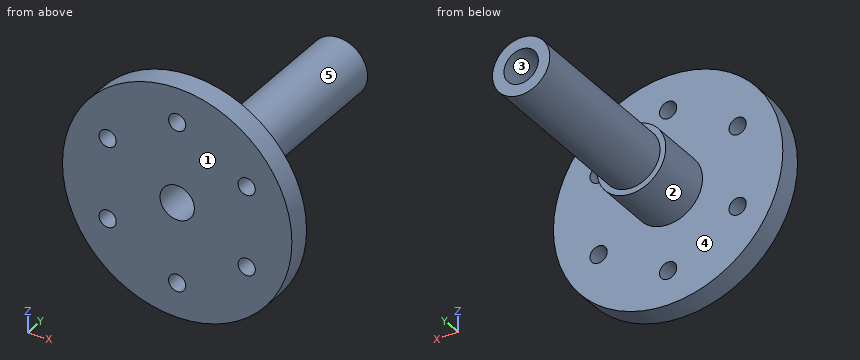
```python
from build123d import *

# Parameters (mm, degrees)
SKETCH_1_R      = 20
SKETCH_1_R_2    = 1.5
SKETCH_1_R_3    = 3
EXTRUDE_1_DEPTH = 4
SKETCH_2_R      = 6
SKETCH_2_R_2    = 3
EXTRUDE_2_DEPTH = 10
SKETCH_3_R      = 5
SKETCH_3_R_2    = 3
EXTRUDE_3_DEPTH = 30


with BuildPart() as part:
    # Sketch 1 → Extrude 1 (new body)
    with BuildSketch(Plane(origin=(0, 0, 0), x_dir=(1, 0, 0), z_dir=(0, 1, 0))):
        with Locations(Location((0, 0, 0), (0, 0, 270))):
            Circle(SKETCH_1_R)
        with Locations(Location((0, 14, 0), (0, 0, 270))):
            Circle(SKETCH_1_R_2, mode=Mode.SUBTRACT)
        with Locations(Location((12.124355653, 7, 0), (0, 0, 270))):
            Circle(SKETCH_1_R_2, mode=Mode.SUBTRACT)
        with Locations(Location((12.124355653, -7, 0), (0, 0, 270))):
            Circle(SKETCH_1_R_2, mode=Mode.SUBTRACT)
        with Locations(Location((0, -14, 0), (0, 0, 270))):
            Circle(SKETCH_1_R_2, mode=Mode.SUBTRACT)
        with Locations(Location((-12.124355653, -7, 0), (0, 0, 270))):
            Circle(SKETCH_1_R_2, mode=Mode.SUBTRACT)
        with Locations(Location((-12.124355653, 7, 0), (0, 0, 270))):
            Circle(SKETCH_1_R_2, mode=Mode.SUBTRACT)
        with Locations(Location((0, 0, 0), (0, 0, 270))):
            Circle(SKETCH_1_R_3, mode=Mode.SUBTRACT)
    extrude(amount=EXTRUDE_1_DEPTH)

    # Sketch 2 → Extrude 2 (add)
    with BuildSketch(Plane(origin=(0, 4, 0), x_dir=(1, 0, 0), z_dir=(0, 1, 0))):
        with Locations(Location((0, 0, 0), (0, 0, 270))):
            Circle(SKETCH_2_R)
        with Locations(Location((0, 0, 0), (0, 0, 270))):
            Circle(SKETCH_2_R_2, mode=Mode.SUBTRACT)
    extrude(amount=EXTRUDE_2_DEPTH)

    # Sketch 3 → Extrude 3 (add)
    with BuildSketch(Plane(origin=(0, 14, 0), x_dir=(1, 0, 0), z_dir=(0, 1, 0))):
        with Locations(Location((0, 0, 0), (0, 0, 270))):
            Circle(SKETCH_3_R)
        with Locations(Location((0, 0, 0), (0, 0, 270))):
            Circle(SKETCH_3_R_2, mode=Mode.SUBTRACT)
    extrude(amount=EXTRUDE_3_DEPTH)


solid = part.part
```
Read the model definition and answer for the solid it produces. Units are mm, in the model's axes. Face numbers are marked on the shaded views. A direction names the side the tool comes from. Coordinates: 2 decimals unless noted, no trailing zeros. Write each loop counter-clockwise with the first axis right and the second up, starting at its lowest first coordinate (ties: lowest second). Pieces come first, ordered by that corner, then holes. Notation, with made-up numbers: (-25.5, 5) - (1.5, 5) arc R35 ccw to (1.5, 44) - close; hole circle Ø1 at (10.25, 16). An arc over 180 degrees is marked (long way). Answer as a JSON object with one key per item and string values. Group by question number.
1. A cutting plane is placed at D-D (y = 7). Determine the outline of the cut face in (x, z), plus the area to 3 significant figures.
2. A cutting plane is placed at C-C (z = -7). Determine the outline of the cut face in (x, y) (3 decimals).
3. Which of the six approach directions +Z, -Z, +X, -X, +Y, -Y give full straight-line access (tool end or side, diameter ignored) to the marked faces 1 and 2?
4. Each of these flat-tipped pins is pushed along its axis until it touches: P1, Ø4, axis at x = -12.12, z = -7, coming from the +Y side; P2, Ø10, axis at y = 6, z = 2, coming from the +X side; P3, Ø2.5, axis at x = 12.12, z = 7, coming from the -Y side (3 decimals); P4, Ø1, axis at x = -4, y = 28, coming from the +Z side. Where does it stop, or does it pass through?
5. A cutting plane is placed at A-A (z = 0). Determine the outline of the cut face in (x, y), plus the area to 3 significant figures.
6. A cutting plane is placed at B-B (x = 0). Determine the outline of the cut face in (y, z), plus the area to 3 significant figures.
7. Consider L1, parallel to X at y = 2.75, z = 7 (3 decimals); L2, parallel to Y at x = -4, z = -9; L3, parallel to Y at x = 5, z = -1. Determine where each line is inside the solid, lowest interval first. Write a range as [from, to].
8. The mould has two halves that part along X. Classify the marked faces 3, 4 and 5: +X half, -X half, draft (parallel to the pull), parting line (faces both ways), or undercut.
Worked out:
{
 "1": {"outline": "circle Ø12 at (0, 0); hole circle Ø6 at (0, 0)", "area": "84.8 mm²"},
 "2": {"outline": "(-18.735, 0) - (-13.624, 0) - (-13.624, 4) - (-18.735, 4) - close; (-10.624, 0) - (10.624, 0) - (10.624, 4) - (-10.624, 4) - close; (13.624, 0) - (18.735, 0) - (18.735, 4) - (13.624, 4) - close"},
 "3": {"face 1": "+Z, -Z, +X, -X, -Y", "face 2": "+Y"},
 "4": {"P1": "stops at y = 4", "P2": "stops at x = 20", "P3": "passes through", "P4": "stops at z = 3.57"},
 "5": {"outline": "(-20, 0) - (-3, 0) - (-3, 44) - (-5, 44) - (-5, 14) - (-6, 14) - (-6, 4) - (-20, 4) - close; (3, 0) - (20, 0) - (20, 4) - (6, 4) - (6, 14) - (5, 14) - (5, 44) - (3, 44) - close", "area": "316 mm²"},
 "6": {"outline": "(0, -20) - (4, -20) - (4, -15.5) - (0, -15.5) - close; (0, -12.5) - (4, -12.5) - (4, -6) - (14, -6) - (14, -5) - (44, -5) - (44, -3) - (0, -3) - close; (0, 3) - (44, 3) - (44, 5) - (14, 5) - (14, 6) - (4, 6) - (4, 12.5) - (0, 12.5) - close; (0, 15.5) - (4, 15.5) - (4, 20) - (0, 20) - close", "area": "292 mm²"},
 "7": {"L1": "x = [-18.735, -13.624], [-10.624, 10.624], [13.624, 18.735]", "L2": "y = [0, 4]", "L3": "y = [0, 14]"},
 "8": {"face 3": "undercut", "face 4": "draft", "face 5": "parting line"}
}
